from build123d import *

# Parameters (mm, degrees)
SKETCH_1_R      = 2.1
EXTRUDE_1_DEPTH = 2


with BuildPart() as part:
    # ｽｹｯﾁ1 → ﾎﾞｽ - 押し出し1 (new body)
    with BuildSketch(Plane.XY):
        Polygon((0, 0), (0, -70), (70, 0), align=None)
        with Locations((10, -40)):
            Circle(SKETCH_1_R, mode=Mode.SUBTRACT)
        with Locations((40, -10)):
            Circle(SKETCH_1_R, mode=Mode.SUBTRACT)
    extrude(amount=EXTRUDE_1_DEPTH)


solid = part.part
Geometry check sheet. Reference: the model listing, model coordinates, mm. Round coordinates to 2 decimals unless told otherwise and drop trailing zeros. Loops run counter-clockwise (first coordinate to the right, second up) from the corner with the lowest first, then second, coordinate; pieces in that order, holes last.
Item 1: Thickness scan on line 1 (X direction, y = -9.5, z = 0.9); line 2 (Y direction, x = 10, z = 0.5); line 3 (Y direction, x = 40, z = 1.1). Record the ranges inside material, lowest first.
Item 2: Mould release check, pull along Y, two halves, no side actions. Record for faces 1 (the flat face through (27, -27, 0)), 2 (the cylindrical face through (9.54, -42.05, 0.99)), 3 (the flat face through (35, -35, 1)): pulls with the +Y half, pulls with the -Y half, needs draft (parallel to the pull), parting line crosses it, or undercut.
Item 3: Cross-section at C-C on z = 0.95. Record the boundary of the cut face in (x, y), then the cut area to 3 significant figures.
Item 4: Cross-section at B-B on y = -40. Record the boundary of the cut face in (x, z).
Item 5: Cross-section at D-D on y = -53. Record the boundary of the cut face in (x, z), then the cut area to 3 significant figures.
Item 6: Cross-section at A-A on x = 40. Record the boundary of the cut face in (y, z).
Item 7: Gauge pin test, flat ends, axial feed: pin 1 (3.5 mm diameter, centred on x = 40, y = -10, fed in from -Z); pin 2 (1 mm diameter, centred on y = -43, z = 1, fed in from +X). Record the tip position at first contact, or that the pin passes through.
Answer sheet:
1. line 1: x = 0 to 37.96, 42.04 to 60.5
1. line 2: y = -60 to -42.1, -37.9 to 0
1. line 3: y = -30 to -12.1, -7.9 to 0
2. face 1: needs draft
2. face 2: undercut
2. face 3: pulls with the -Y half
3. outline: (0, -70) - (70, 0) - (0, 0) - close; hole circle Ø4.2 at (10, -40); hole circle Ø4.2 at (40, -10)
3. area: 2,420 mm2
4. outline: (0, 0) - (7.9, 0) - (7.9, 2) - (0, 2) - close; (12.1, 0) - (30, 0) - (30, 2) - (12.1, 2) - close
5. outline: (0, 0) - (17, 0) - (17, 2) - (0, 2) - close
5. area: 34.0 mm2
6. outline: (-30, 0) - (-12.1, 0) - (-12.1, 2) - (-30, 2) - close; (-7.9, 0) - (0, 0) - (0, 2) - (-7.9, 2) - close
7. pin 1: passes through
7. pin 2: stops at x = 27.5
